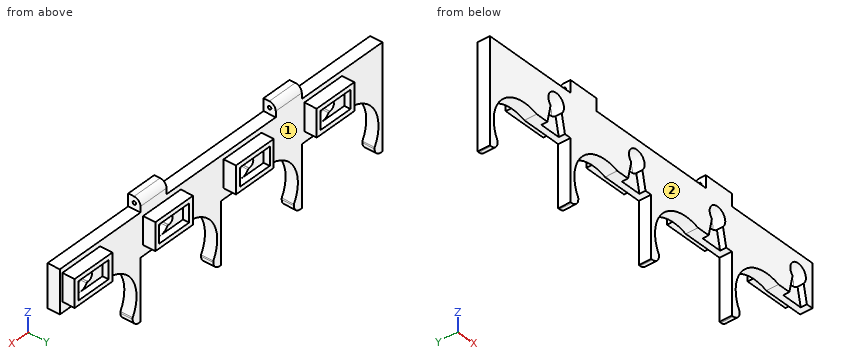
```python
from build123d import *

# Parameters (mm, degrees)
ESQUISSE1_R                = 6
BOSS_EXTRU_1_DEPTH         = 8
ESQUISSE2_W                = 29
ESQUISSE2_H                = 18
BOSS_EXTRU_2_DEPTH         = 4
ESQUISSE3_W                = 29
ESQUISSE3_H                = 18
ESQUISSE3_W_2              = 23
ESQUISSE3_H_2              = 12
BOSS_EXTRU_3_DEPTH         = 4
ENL_V_MAT_EXTRU_1_DEPTH    = 4
R_P_TITION_LIN_AIRE1_COUNT = 4
R_P_TITION_LIN_AIRE1_PITCH = 62
ESQUISSE5_R                = 1.1
BOSS_EXTRU_4_DEPTH         = 20


with BuildPart() as part:
    # Esquisse1 → Boss.-Extru.1 (new body)
    with BuildSketch(Plane(origin=(0, 0, 0), x_dir=(1, 0, 0), z_dir=(0, 1, 0))):
        with BuildLine():
            Line((0, 0), (6, 0))
            Line((6, 0), (36, 0))
            Line((36, 0), (62, 0))
            Line((62, 0), (62, 28.055987731))
            Line((62, 28.055987731), (36, 28.055987731))
            ThreePointArc((36, 28.055987731), (9.034681758, 34.39083629), (6, 61.923533231))
            Line((6, 61.923533231), (6, 62.923533231))
            ThreePointArc((6, 62.923533231), (4.535533906, 66.459067137), (1, 67.923533231))
            Line((1, 67.923533231), (0, 67.923533231))
            Line((0, 67.923533231), (0, 0))
        make_face()
        with Locations((51, 12.304583192)):
            Circle(ESQUISSE1_R, mode=Mode.SUBTRACT)
    extrude(amount=BOSS_EXTRU_1_DEPTH)

    # Esquisse2 → Boss.-Extru.2 (add)
    with BuildSketch(Plane(origin=(0, 8, 0), x_dir=(1, 0, 0), z_dir=(0, 1, 0))):
        with Locations((45.5, 12.304583192)):
            Rectangle(ESQUISSE2_W, ESQUISSE2_H)
        with BuildLine():
            Line((45, 15.304583192), (45.255437353, 15.304583192))
            ThreePointArc((45.255437353, 15.304583192), (45.718347403, 15.418177932), (46.07608916, 15.733154621))
            ThreePointArc((46.07608916, 15.733154621), (57, 12.304583192), (46.07608916, 8.876011764))
            ThreePointArc((46.07608916, 8.876011764), (45.718347403, 9.190988453), (45.255437353, 9.304583192))
            Line((45.255437353, 9.304583192), (45, 9.304583192))
            ThreePointArc((45, 9.304583192), (42, 12.304583192), (45, 15.304583192))
        make_face(mode=Mode.SUBTRACT)
    extrude(amount=BOSS_EXTRU_2_DEPTH)

    # Esquisse3 → Boss.-Extru.3 (add)
    with BuildSketch(Plane(origin=(0, 12, 0), x_dir=(1, 0, 0), z_dir=(0, 1, 0))):
        with Locations((45.5, 12.304583192)):
            Rectangle(ESQUISSE3_W, ESQUISSE3_H)
        with Locations((45.5, 12.304583192)):
            Rectangle(ESQUISSE3_W_2, ESQUISSE3_H_2, mode=Mode.SUBTRACT)
    extrude(amount=BOSS_EXTRU_3_DEPTH)

    # Esquisse4 → Enlèv. mat.-Extru.1 (cut)
    with BuildSketch(Plane.XZ):
        Polygon((47.7, -17.055987731), (54.3, -17.055987731), (55.193703609, -16.162284122), (57.721788353, -28.055987731), (54.3, -28.055987731), (47.7, -28.055987731), (44.278211647, -28.055987731), (46.806296391, -16.162284122), align=None)
    extrude(amount=-ENL_V_MAT_EXTRU_1_DEPTH, mode=Mode.SUBTRACT)

    # Répétition linéaire1: part ×4


with BuildPart() as part_1:
    add(part.part)
    with Locations(*[(i * R_P_TITION_LIN_AIRE1_PITCH, 0, 0) for i in range(1, R_P_TITION_LIN_AIRE1_COUNT)]):
        add(part.part)

    # Esquisse5 → Boss.-Extru.4 (add)
    with BuildSketch(Plane.ZY.offset(-62)):
        with BuildLine():
            Line((0, 8), (3.8, 8))
            ThreePointArc((3.8, 8), (6.769848481, 6.769848481), (8, 3.8))
            Line((8, 3.8), (8, 0))
            Line((8, 0), (0, 0))
            Line((0, 0), (0, 8))
        make_face()
        with Locations((4, 4)):
            Circle(ESQUISSE5_R, mode=Mode.SUBTRACT)
    boss_extru_4 = extrude(amount=-BOSS_EXTRU_4_DEPTH)

    # Symétrie1: Boss.-Extru.4 across plane
    add(boss_extru_4.mirror(Plane(origin=(124, 8, 0), x_dir=(0, 0, 1), z_dir=(1, 0, 0))))


solid = part_1.part
```
For this review, take the finished solid that the model builds, in its own axes (mm). Face numbers are marked on the shaded views. Give positions to 0.01 mm unless a question says otherwise; leave off trailing zeros. Order: outer loops, then holes, each group sorted by start corner. A loop starts at its lowest first (then second) coordinate and runs counter-clockwise, first axis right, second up.
1) The part is to be moulded in two halves that separate along X. For the marked faces 1 and 2, say which applies: released by +X, released by -X, zero draft, split by the parting line, or undercut.
2) Take a section at C-C (x = 197.5). Give the boundary of the cut face in (y, z), then the cut area to 3 significant figures.
3) Take a section at A-A (z = -40.5). Give the boundary of the cut face in (x, y), then the cut area to 3 significant figures.
4) Insertion check: pin 1 (1.2 mm diameter, centred on x = 113, y = 13.5, fed in from +Z); pin 2 (5 mm diameter, centred on x = 116, z = -14.5, fed in from +Y); pin 3 (3 mm diameter, centred on y = 4, z = 4, fed in from +X). Each pin has a flat end and moves straight along its axis. Give the tip position at first contact, or say it passes through.
5) Take a section at B-B (z = -59). Give the boundary of the cut face in (x, y), then the cut area to 3 significant figures.
6) Wall thickness on line 1 (X direction, y = 13, z = -18.5); line 2 (X direction, y = 7.5, z = -34); line 3 (Z direction, x = 113, y = 9.45): over which ranges is each line inside the solid? List them lowest first.
7) Take a section at D-D (x = 137.5). Give the boundary of the cut face in (y, z), then the cut area to 3 significant figures.
Derived:
1. face 1: undercut
1. face 2: zero draft
2. outline: (0, -31.98) - (8, -31.98) - (8, 0) - (0, 0) - close
2. area: 256 mm2
3. outline: (0, 0) - (5.09, 0) - (5.09, 8) - (0, 8) - close; (62, 0) - (67.09, 0) - (67.09, 8) - (62, 8) - close; (124, 0) - (129.09, 0) - (129.09, 8) - (124, 8) - close; (186, 0) - (191.09, 0) - (191.09, 8) - (186, 8) - close
3. area: 163 mm2
4. pin 1: stops at z = -3.3
4. pin 2: stops at y = 12
4. pin 3: stops at x = 186
5. outline: (0, 0) - (4.63, 0) - (4.63, 8) - (0, 8) - close; (62, 0) - (66.63, 0) - (66.63, 8) - (62, 8) - close; (124, 0) - (128.63, 0) - (128.63, 8) - (124, 8) - close; (186, 0) - (190.63, 0) - (190.63, 8) - (186, 8) - close
5. area: 148 mm2
6. line 1: x = 31 to 60, 93 to 122, 155 to 184, 217 to 246
6. line 2: x = 0 to 9.39, 62 to 71.39, 124 to 133.39, 186 to 195.39
6. line 3: z = -21.3 to -18.3, -6.3 to -3.3
7. outline: (0, -30.46) - (8, -30.46) - (8, 0) - (0, 0) - close
7. area: 244 mm2
